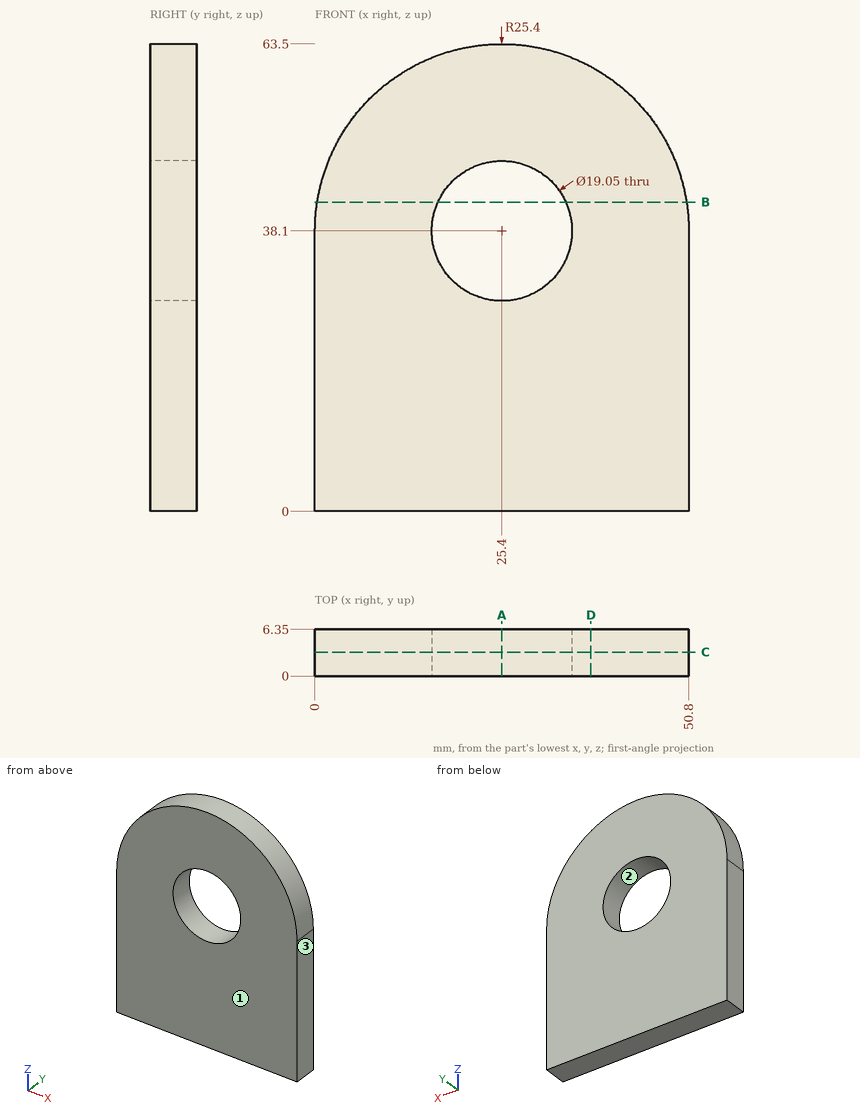
Part print with two shaded views. Sizes in mm from the minimum x, y, z corner. Give positions to 0.01 mm unless a question says otherwise; leave off trailing zeros. Order: outer loops, then holes, each group sorted by start corner. A loop starts at its lowest first (then second) coordinate and runs counter-clockwise, first axis right, second up.
(1) Drill centre lines: L1, parallel to Z at x = 25.4, y = 3.75 (3 decimals); L2, parallel to X at y = 4, z = 38.1 (3 decimals); L3, parallel to Z at x = 30, y = 1.5. Where is each one in solid material? Low to high.
(2) Saw through at D-D, the plane x = 37.5. Give the cut face in (y, z), then the cut area to 3 significant figures.
(3) Saw through at B-B, the plane z = 42. Give the cut face in (x, y), then the cut area to 3 significant figures.
(4) Flat gauge pin, fed straight in: pin 1 (3 mm diameter, centred on x = 18.5, y = 5.5, fed in from +Z). Where does the tip first touch, or does it go through?
(5) Saw through at A-A, the plane x = 25.4. Give the cut face in (y, z) (3 decimals).
(6) Saw through at C-C, the plane y = 3.25. Give the cut face in (x, z) (3 decimals).
(7) Mould opens along X. For the marked faces 1, 2 and 3 say: released by +X, released by -X, zero draft, split by the parting line, or undercut.
Results found:
1. L1: z = 0 to 28.575, 47.625 to 63.5
1. L2: x = 0 to 15.875, 34.925 to 50.8
1. L3: z = 0 to 29.76, 46.44 to 63.08
2. outline: (0, 0) - (6.35, 0) - (6.35, 60.43) - (0, 60.43) - close
2. area: 384 mm2
3. outline: (0.3, 0) - (16.71, 0) - (16.71, 6.35) - (0.3, 6.35) - close; (34.09, 0) - (50.5, 0) - (50.5, 6.35) - (34.09, 6.35) - close
3. area: 208 mm2
4. pin 1: stops at z = 62.92
5. outline: (0, 0) - (6.35, 0) - (6.35, 28.575) - (0, 28.575) - close; (0, 47.625) - (6.35, 47.625) - (6.35, 63.5) - (0, 63.5) - close
6. outline: (0, 0) - (50.8, 0) - (50.8, 38.1) arc R25.4 ccw to (0, 38.1) - close; hole circle Ø19.05 at (25.4, 38.1)
7. face 1: zero draft
7. face 2: undercut
7. face 3: released by +X
